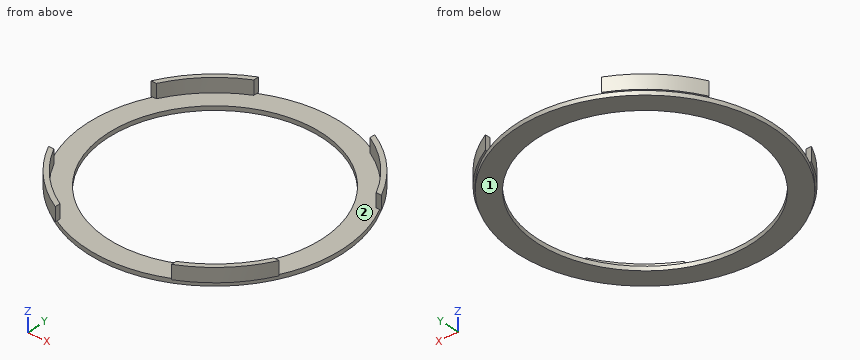
from build123d import *

# Parameters (mm, degrees)
F0_R      = 54.8
F1_DEPTH  = 1.8
F2_R      = 55.5
F3_DEPTH  = 6
F4_W      = 50
F4_H      = 125
F5_DEPTH  = 6
F6_W      = 120
F6_H      = 50
F7_DEPTH  = 6
F8_R      = 53.5
F9_DEPTH  = 6
F10_R     = 46
F11_DEPTH = 25


with BuildPart() as f1:
    # F0 (on Top) → F1 (new body)
    with BuildSketch(Plane.XY):
        Circle(F0_R)
    extrude(amount=F1_DEPTH)

    # F2 (on face) → F3 (join)
    with BuildSketch(Plane.XY.offset(1.8)):
        Circle(F2_R)
    extrude(amount=F3_DEPTH)

    # F4 (on face) → F5 (cut)
    with BuildSketch(Plane.XY.offset(7.8)):
        Rectangle(F4_W, F4_H)
    extrude(amount=-F5_DEPTH, mode=Mode.SUBTRACT)

    # F6 (on face) → F7 (cut)
    with BuildSketch(Plane.XY.offset(7.8)):
        Rectangle(F6_W, F6_H)
    extrude(amount=-F7_DEPTH, mode=Mode.SUBTRACT)

    # F8 (on face) → F9 (cut)
    with BuildSketch(Plane.XY.offset(7.8)):
        Circle(F8_R)
    extrude(amount=-F9_DEPTH, mode=Mode.SUBTRACT)

    # F10 (on face) → F11 (cut)
    with BuildSketch(Plane.XY.offset(1.8)):
        Circle(F10_R)
    extrude(amount=-F11_DEPTH, mode=Mode.SUBTRACT)


solid = f1.part
The listing builds one solid part. Answer for the finished solid, in the listing's coordinates (mm). Face numbers are marked on the shaded views. Give positions to 0.01 mm unless a question says otherwise; leave off trailing zeros. Write each loop counter-clockwise with the first axis right and the second up, starting at its lowest first coordinate (ties: lowest second). Pieces come first, ordered by that corner, then holes. Notation, with made-up numbers: (2, -38) -> (30, -38) arc R33 cw to (30, 1) -> close; hole circle Ø5 at (68.25, 2.25). An arc over 180 degrees is marked (long way). Use a Markdown table: item, result.
(1) Section D-D, the plane y = 29 is taken. Determine the outline of the cut face in (x, z).
Return value:
| item | result |
|---|---|
| outline | (-47.32, 1.8) -> (-46.5, 1.8) -> (-46.5, 0) -> (-35.71, 0) -> (-35.71, 1.8) -> (-44.96, 1.8) -> (-44.96, 7.8) -> (-47.32, 7.8) -> close; (35.71, 0) -> (46.5, 0) -> (46.5, 1.8) -> (47.32, 1.8) -> (47.32, 7.8) -> (44.96, 7.8) -> (44.96, 1.8) -> (35.71, 1.8) -> close |
(2) Section A-A, the plane y = 0 is taken. Determine the outline of the cut face in (x, z).
Return value:
| item | result |
|---|---|
| outline | (-54.8, 0) -> (-46, 0) -> (-46, 1.8) -> (-54.8, 1.8) -> close; (46, 0) -> (54.8, 0) -> (54.8, 1.8) -> (46, 1.8) -> close |
(3) Section B-B, the plane z = 4.75 is taken. Determine the outline of the cut face in (x, y), then the cut area to 3 significant figures.
Return value:
| item | result |
|---|---|
| outline | (-49.55, -25) arc R55.5 ccw to (-25, -49.55) -> (-25, -47.3) arc R53.5 cw to (-47.3, -25) -> close; (-49.55, 25) -> (-47.3, 25) arc R53.5 cw to (-25, 47.3) -> (-25, 49.55) arc R55.5 ccw to start; (25, -49.55) arc R55.5 ccw to (49.55, -25) -> (47.3, -25) arc R53.5 cw to (25, -47.3) -> close; (25, 47.3) arc R53.5 cw to (47.3, 25) -> (49.55, 25) arc R55.5 ccw to (25, 49.55) -> close |
| area | 269 mm2 |
(4) Determine the mould class of the marked faces 1 and 2 for opening direction Y: released by +Y, released by -Y, zero draft, split by the parting line, or undercut.
Return value:
| item | result |
|---|---|
| face 1 | zero draft |
| face 2 | undercut |
(5) Find the intervals of material crossed by probe 1 along Y at (x, z) = (0, 0.6); probe 2 along Z at (x, y) = (-12.5, 49.5); probe 3 along Y at (x, z) = (35, 4.75), in increasing order. Write a range as from..to.
Return value:
| item | result |
|---|---|
| probe 1 | -54.8..-46, 46..54.8 |
| probe 2 | 0..1.8 |
| probe 3 | -43.07..-40.46, 40.46..43.07 |
(6) Flat-ended cylindrical pins translate along their axes: P1, Ø2.5, axis at x = -48, z = 4.5, coming from the -Y side; P2, Ø1, axis at y = 23.5, z = 6.5, coming from the -X side; P3, Ø0.7, axis at y = -48, z = 4, coming from the -X side; P4, Ø0.7, axis at y = 48.5, z = 5.5, coming from the -X side. Find the tip coordinate at first contact, or state that the pin passes through.
Return value:
| item | result |
|---|---|
| P1 | y = -29.91 |
| P2 | through |
| P3 | x = -28.46 |
| P4 | x = -27.6 |
